Geometry: final body of the model. Coordinates: model frame, mm. Round coordinates to 2 decimals unless told otherwise and drop trailing zeros. Loops run counter-clockwise (first coordinate to the right, second up) from the corner with the lowest first, then second, coordinate; pieces in that order, holes last. Notation, with made-up numbers: (0.25, -27.75) -> (48.25, -27.75) arc R12 cw to (48.25, -13.75) -> close; hole circle Ø6 at (40.5, 60.5). An arc over 180 degrees is marked (long way). Answer in a Markdown table with one row per item.
```python
from build123d import *

# Parameters (mm, degrees)
F1_DEPTH = 12.7
F3_DEPTH = 50.8


# Not quite as in the source:
# - a feature names something its author has since deleted; it is built from what else it names


with BuildPart() as f1:
    # F0 (on Front) → F1 (new body)
    with BuildSketch(Plane.XZ):
        with BuildLine():
            ThreePointArc((-95.1022987413, 273.3746719669), (60.4202481719, 242.4393139794), (192.265897133, 154.3428678411))
            Line((192.265897133, 154.3428678411), (412.2821720991, 374.3591428073))
            ThreePointArc((412.2821720992, 374.3591428073), (-95.1022987413, 584.5246719669), (-602.4867695817, 374.3591428072))
            Line((-602.4867695817, 374.3591428073), (-382.4704946155, 154.3428678411))
            ThreePointArc((-382.4704946155, 154.3428678411), (-250.6248456544, 242.4393139794), (-95.1022987413, 273.3746719669))
        make_face()
        with BuildLine():
            ThreePointArc((-525.7952385086, 333.5886362184), (-338.1062782931, 453.6381751115), (-120.5022987413, 501.4664686041))
            Line((-120.5022987413, 501.4664686041), (-120.5022987413, 336.1876832954))
            ThreePointArc((-120.5022987413, 336.1876832954), (-274.9252436096, 301.1056642939), (-408.9254886305, 216.7188863404))
            Line((-408.9254886305, 216.7188863404), (-525.7952385086, 333.5886362184))
        make_face(mode=Mode.SUBTRACT)
        with BuildLine():
            Line((-69.7022987413, 336.1876832954), (-69.7022987413, 501.4664686041))
            ThreePointArc((-69.7022987413, 501.4664686041), (147.9016808106, 453.6381751115), (335.5906410261, 333.5886362184))
            Line((335.5906410261, 333.5886362184), (218.720891148, 216.7188863404))
            ThreePointArc((218.720891148, 216.7188863404), (84.7206461271, 301.1056642939), (-69.7022987413, 336.1876832954))
        make_face(mode=Mode.SUBTRACT)
        with BuildLine():
            ThreePointArc((192.265897133, 154.3428678411), (280.3623432713, 22.49721888), (311.2977012587, -133.0253280331))
            ThreePointArc((311.2977012587, -133.0253280331), (-250.6248456544, -508.4899700457), (-382.4704946155, 154.3428678411))
            Line((-382.4704946155, 154.3428678411), (-602.4867695817, 374.3591428073))
            ThreePointArc((-602.4867695817, 374.3591428072), (-758.0320572947, 141.5691688604), (-812.6522987413, -133.0253280331))
            Line((-812.6522987413, -133.0253280331), (-812.6522987413, -844.2450938398))
            Line((-812.6522987413, -844.2450938398), (0, -844.2450938398))
            Line((0, -844.2450938398), (622.4477012587, -844.2450938398))
            Line((622.4477012587, -844.2450938398), (622.4477012587, -133.0253280331))
            ThreePointArc((622.4477012587, -133.0253280331), (567.8274598122, 141.5691688604), (412.2821720992, 374.3591428073))
            Line((412.2821720991, 374.3591428073), (192.265897133, 154.3428678411))
        make_face()
        with BuildLine():
            ThreePointArc((-444.8465131148, 180.7978618561), (-533.9364452785, 34.9943191303), (-565.0022987413, -133.0253280331))
            Line((-565.0022987413, -133.0253280331), (-730.1022987413, -133.0253280331))
            ThreePointArc((-730.1022987413, -133.0253280331), (-686.5094627576, 98.1944080408), (-561.7162629929, 297.6676117342))
            Line((-561.7162629929, 297.6676117342), (-444.8465131148, 180.7978618561))
        make_face(mode=Mode.SUBTRACT)
        with BuildLine():
            ThreePointArc((371.5116655103, 297.6676117342), (496.3048652751, 98.1944080408), (539.8977012587, -133.0253280331))
            Line((539.8977012587, -133.0253280331), (374.7977012587, -133.0253280331))
            ThreePointArc((374.7977012587, -133.0253280331), (343.731847796, 34.9943191303), (254.6419156323, 180.7978618561))
            Line((254.6419156323, 180.7978618561), (371.5116655103, 297.6676117342))
        make_face(mode=Mode.SUBTRACT)
    extrude(amount=F1_DEPTH)

    # F2 (on face) → F3 (join)
    with BuildSketch(Plane.XZ.offset(12.7)):
        Polygon((-691.485961068, 86.5121113929), (-681.7658018859, 109.9786515187), (-672.0456427039, 133.4451916445), (-718.9787229554, 152.8855100086), (-738.4190413196, 105.952429757), align=None)
        Polygon((528.7741254729, 152.8855100086), (481.8410452213, 133.4451916445), (491.5612025764, 109.9786559296), (501.2813635855, 86.5121113929), (548.2144438371, 105.952429757), align=None)
        Polygon((-381.013136783, 490.851096181), (-361.5728184189, 443.9180159294), (-338.1062857272, 453.6381720322), (-314.6397381673, 463.3583342936), (-334.0800565315, 510.2914145452), align=None)
        Polygon((143.8754590489, 510.2914145452), (124.4351406848, 463.3583342936), (147.9016748411, 453.6381775841), (171.3682209364, 443.9180159294), (190.8085393005, 490.851096181), align=None)
    extrude(amount=F3_DEPTH)


solid = f1.part
```
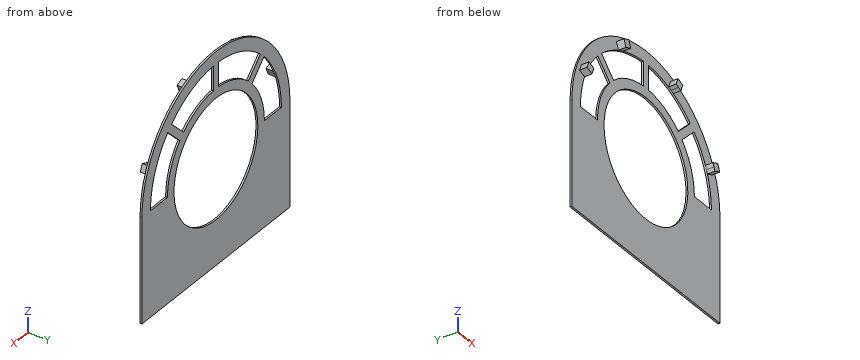
Item 1: Section query B-B, the plane y = -37. Output: boundary loops of the cut face in (x, z), and give its area (3 significant figures).
Ans:
| item | result |
|---|---|
| outline | (-738.42, 105.95) -> (-691.49, 86.51) -> (-672.05, 133.45) -> (-718.98, 152.89) -> close; (-381.01, 490.85) -> (-361.57, 443.92) -> (-314.64, 463.36) -> (-334.08, 510.29) -> close; (124.44, 463.36) -> (171.37, 443.92) -> (190.81, 490.85) -> (143.88, 510.29) -> close; (481.84, 133.45) -> (501.28, 86.51) -> (548.21, 105.95) -> (528.77, 152.89) -> close |
| area | 10,300 mm2 |
Item 2: Section query C-C, the plane x = 433. Output: boundary loops of the cut face in (y, z), and give its area (3 significant figures).
Ans:
| item | result |
|---|---|
| outline | (-12.7, -844.25) -> (0, -844.25) -> (0, -133.03) -> (-12.7, -133.03) -> close; (-12.7, 219.58) -> (0, 219.58) -> (0, 352.76) -> (-12.7, 352.76) -> close |
| area | 10,700 mm2 |
Item 3: Section query A-A, the plane z = -83. Output: boundary loops of the cut face in (x, y), and give its area (3 significant figures).
Ans:
| item | result |
|---|---|
| outline | (-810.91, -12.7) -> (-728.13, -12.7) -> (-728.13, 0) -> (-810.91, 0) -> close; (-562.33, -12.7) -> (-498.41, -12.7) -> (-498.41, 0) -> (-562.33, 0) -> close; (308.21, -12.7) -> (372.13, -12.7) -> (372.13, 0) -> (308.21, 0) -> close; (537.92, -12.7) -> (620.7, -12.7) -> (620.7, 0) -> (537.92, 0) -> close |
| area | 3,730 mm2 |
Item 4: Ray query, L1, parallel to Z at x = -416, y = -12; L2, parallel to Y at x = -373.5, z = 240.5; L3, parallel to X at y = -38, z = 479.5. Return the intervals inside material, ascending.
Ans:
| item | result |
|---|---|
| L1 | -844.25 to -382.4, 116.35 to 223.79, 414.93 to 508.77 |
| L2 | -12.7 to 0 |
| L3 | -376.31 to -321.33, 131.12 to 186.11 |
Item 5: Section query D-D, the plane z = -247. Output: boundary loops of the cut face in (x, y).
Ans:
| item | result |
|---|---|
| outline | (-812.65, -12.7) -> (-485.19, -12.7) -> (-485.19, 0) -> (-812.65, 0) -> close; (294.99, -12.7) -> (622.45, -12.7) -> (622.45, 0) -> (294.99, 0) -> close |
Item 6: First-contact query: P1, Ø14, axis at y = -6, z = 383, coming from the +X side; P2, Ø4, axis at x = -685.5, y = -7.5, coming from the +Z side; P3, Ø5, axis at x = 165, z = 243.5, coming from the +Y side; P4, Ø10, axis at y = -8.5, z = 415.5, coming from the -X side. Flat tips, straight axial feed; report the tip coordinate or a pass-through.
Ans:
| item | result |
|---|---|
| P1 | x = 410.64 |
| P2 | z = 277.66 |
| P3 | y = 0 |
| P4 | x = -563.57 |
